Read the model definition and answer for the solid it produces. Units are mm, in the model's axes. Round coordinates to 2 decimals unless told otherwise and drop trailing zeros. Write each loop counter-clockwise with the first axis right and the second up, starting at its lowest first coordinate (ties: lowest second). Pieces come first, ordered by that corner, then holes. Notation, with made-up numbers: (45, 74) -> (67, 74) arc R28 cw to (67, 99) -> close; hole circle Ø6 at (-8.75, -16). An arc over 180 degrees is marked (long way). Return JSON: item names as keys, results as strings. Group by question number.
(1) Given pin 1 (1.5 mm diameter, centred on x = 6, z = 116.5, fed in from +Y), flat-ended and moving along its own axis, determine where the tip first touches the part or whether it passes through.
(2) A cutting plane is placed at A-A on y = -0.7. Give the vertices of the cut face in (x, z), then the cut area to 3 significant figures.
(3) Straight lines are drawn through the part: line 1 (X direction, y = -0.55, z = 185); line 2 (X direction, y = -0.2, z = 15.5); line 3 (Z direction, x = 7, y = -1.6). For each, find the intervals that lie inside material, in ascending order.
(4) A cutting plane is placed at B-B on z = 44.5. Give the vertices of the cut face in (x, y), then the cut area to 3 significant figures.
(5) The mould has two halves that part along Z. Classify faces 1 (the flat face through (8, -2, 101)), 2 (the cylindrical face through (9.61, -0.99, 157.53)): released by +Z, released by -Z, zero draft, split by the parting line, or undercut.
(6) A cutting plane is placed at C-C on x = 7.75. Give the vertices of the cut face in (y, z).
```python
from build123d import *

# Parameters (mm, degrees)
F0_W     = 16
F0_H     = 200
F0_R     = 3
F1_DEPTH = 2


with BuildPart() as f1:
    # F0 (on Front) → F1 (new body)
    with BuildSketch(Plane.XZ):
        with Locations((8, 100)):
            Rectangle(F0_W, F0_H)
        with BuildLine():
            Line((4.5, 15), (4.5, 95))
            ThreePointArc((4.5, 95), (7.5, 98), (10.5, 95))
            Line((10.5, 95), (10.5, 15))
            ThreePointArc((10.5, 15), (7.5, 12), (4.5, 15))
        make_face(mode=Mode.SUBTRACT)
        with Locations((8, 155)):
            Circle(F0_R, mode=Mode.SUBTRACT)
        with Locations((8, 185)):
            Circle(F0_R, mode=Mode.SUBTRACT)
    extrude(amount=F1_DEPTH)


solid = f1.part
```
Checks:
{
 "1": {"pin 1": "stops at y = 0"},
 "2": {"outline": "(0, 0) -> (16, 0) -> (16, 200) -> (0, 200) -> close; hole (4.5, 15) arc R3 ccw to (10.5, 15) -> (10.5, 95) arc R3 ccw to (4.5, 95) -> close; hole circle Ø6 at (8, 155); hole circle Ø6 at (8, 185)", "area": "2,640 mm^2"},
 "3": {"line 1": "x = 0 to 5, 11 to 16", "line 2": "x = 0 to 4.5, 10.5 to 16", "line 3": "z = 0 to 12.04, 97.96 to 152.17, 157.83 to 182.17, 187.83 to 200"},
 "4": {"outline": "(0, -2) -> (4.5, -2) -> (4.5, 0) -> (0, 0) -> close; (10.5, -2) -> (16, -2) -> (16, 0) -> (10.5, 0) -> close", "area": "20.0 mm^2"},
 "5": {"face 1": "zero draft", "face 2": "undercut"},
 "6": {"outline": "(-2, 0) -> (0, 0) -> (0, 12.01) -> (-2, 12.01) -> close; (-2, 97.99) -> (0, 97.99) -> (0, 152.01) -> (-2, 152.01) -> close; (-2, 157.99) -> (0, 157.99) -> (0, 182.01) -> (-2, 182.01) -> close; (-2, 187.99) -> (0, 187.99) -> (0, 200) -> (-2, 200) -> close"}
}
